Part model, mm, in its own coordinate system. A direction names the side the tool comes from. Coordinates: 2 decimals unless noted, no trailing zeros. Order: outer loops, then holes, each group sorted by start corner. A loop starts at its lowest first (then second) coordinate and runs counter-clockwise, first axis right, second up.
1) Cut at B-B (x = 0). List the corners of the cut face in (y, z).
2) Cut at C-C (y = 13.5). List the corners of the cut face in (x, z), and give its area (3 significant figures).
3) Wall check: L1, parallel to X at y = -3.3, z = 0; L2, parallel to Z at x = 7.5, y = -1.05; L3, parallel to Y at x = 9, z = 2.75. Give the ranges that are in metal, low to high.
4) Tool access for faces 4 (the cylindrical face through (1.43, -45.14, -2.75)), 5 (the flat face through (7.66, -45.87, 1.51)), 6 (the flat face through (0, 10, -1.5)), 7 (the cylindrical face through (6.25, -2.46, -0.05)): list every direction of +Z, -Z, +X, -X, +Y, -Y with a clear straight run to the whole face (end or side of a thin tool).
5) Cut at D-D (z = -5.25). List the corners of the cut face in (x, y).
6) Mould opens along X. For faces 1 (the cylindrical face through (0, -49, -1)), 2 (the flat face through (-7.53, -45.875, -1.783)), 3 (the cylindrical face through (10.2, -31.4, -0.1)) say: +X half, -X half, draft (parallel to the pull), parting line (faces both ways), or undercut.
7) Pin check, flat tips, straight feed: pin 1 Ø3 at (x, z) = (7.5, 0) entering from -Y; pin 2 Ø10.5 at (x, y) = (3, -28) entering from -Z; pin 3 Ø6 at (x, z) = (-5, -6) entering from -Y; pin 4 Ø6 at (x, z) = (4.5, -2) entering from +Y. Stop position of each tip, or through.
```python
from build123d import *

# Parameters (mm, degrees)
SKETCH_R              = 10
PAD_DEPTH             = 19
SKETCH001_R           = 3.5
PAD001_DEPTH          = 3
SKETCH002_R           = 2
PAD002_DEPTH          = 14.5
SKETCH003_W           = 10
SKETCH003_H           = 5
POCKET_DEPTH          = 14.5
PAD003_DEPTH          = 25.1
SKETCH005_R           = 3.1
PAD004_DEPTH          = 2.1
SKETCH006_R           = 1
PAD005_DEPTH          = 6
PAD006_DEPTH          = 3.6
SKETCH009_R           = 0.5
POCKET001_DEPTH       = 5
POLARPATTERN_COUNT    = 2
POLARPATTERN001_COUNT = 2
SKETCH010_R           = 1.25
POCKET002_DEPTH       = 5


with BuildPart() as part:
    # Sketch → Pad (new body)
    with BuildSketch(Plane.XZ):
        Circle(SKETCH_R)
    extrude(amount=PAD_DEPTH)

    # Sketch001 (on Face2 of Pad) → Pad001 (join)
    with BuildSketch(Plane(origin=(0, 0, 0), x_dir=(1, 0, 0), z_dir=(0, 1, 0))):
        Circle(SKETCH001_R)
    extrude(amount=PAD001_DEPTH)

    # Sketch002 (on Face5 of Pad001) → Pad002 (join)
    with BuildSketch(Plane(origin=(0, 3, 0), x_dir=(1, 0, 0), z_dir=(0, 1, 0))):
        Circle(SKETCH002_R)
    extrude(amount=PAD002_DEPTH)

    # Sketch003 (on Face7 of Pad002) → Pocket (cut)
    with BuildSketch(Plane(origin=(0, 17.5, 0), x_dir=(1, 0, 0), z_dir=(0, 1, 0))):
        with Locations((0, 4)):
            Rectangle(SKETCH003_W, SKETCH003_H)
    extrude(amount=-POCKET_DEPTH, mode=Mode.SUBTRACT)

    # Sketch004 (on Face3 of Pocket) → Pad003 (join)
    with BuildSketch(Plane.XZ.offset(19)):
        with BuildLine():
            Line((-6.689544, 7.7), (6.689544, 7.7))
            ThreePointArc((6.689544, -7.7), (10.2, 0), (6.689544, 7.7))
            Line((6.689544, -7.7), (-6.689544, -7.7))
            ThreePointArc((-6.689544, 7.7), (-10.2, 0), (-6.689544, -7.7))
        make_face()
    extrude(amount=PAD003_DEPTH)

    # Sketch005 (on Face14 of Pad003) → Pad004 (join)
    with BuildSketch(Plane.XZ.offset(44.1)):
        Circle(SKETCH005_R)
    extrude(amount=PAD004_DEPTH)

    # Sketch006 (on Face21 of Pad004) → Pad005 (join)
    with BuildSketch(Plane.XZ.offset(46.2)):
        Circle(SKETCH006_R)
    extrude(amount=PAD005_DEPTH)

    # Sketch008 (on Face14 of Pad005) → Pad006 (join)
    with BuildSketch(Plane.XZ.offset(44.1)):
        Polygon((6.603759, 1.445812), (8.483144, 2.129852), (8.58575, 1.847944), (6.706365, 1.163904), align=None)
    pad006 = extrude(amount=PAD006_DEPTH)

    # Sketch009 (on Face21 of Pad006) → Pocket001 (cut)
    with BuildSketch(Plane(origin=(0.410424, 0, -1.127631), x_dir=(0.939693, 0, 0.34202), z_dir=(0.34202, 0, -0.939693))):
        with Locations((7.689708, 46.695641)):
            Circle(SKETCH009_R)
    pocket001 = extrude(amount=-POCKET001_DEPTH, mode=Mode.SUBTRACT)

    # PolarPattern: Pad006 ×2 about axis
    polarpattern_axis = Axis((0, -44.1, 0), (0, -1, 0))
    for i in range(1, POLARPATTERN_COUNT):
        add(pad006.rotate(polarpattern_axis, i * 360 / POLARPATTERN_COUNT))

    # PolarPattern001: Pocket001 ×2 about axis
    polarpattern001_axis = Axis((0, 0, 0), (0, 1, 0))
    for i in range(1, POLARPATTERN001_COUNT):
        add(pocket001.rotate(polarpattern001_axis, i * 360 / POLARPATTERN001_COUNT), mode=Mode.SUBTRACT)

    # Sketch010 (on Face2 of PolarPattern001) → Pocket002 (cut)
    with BuildSketch(Plane(origin=(0, 0, 0), x_dir=(1, 0, 0), z_dir=(0, 1, 0))):
        with Locations((7.5, 0)):
            Circle(SKETCH010_R)
        with Locations((-7.5, 0)):
            Circle(SKETCH010_R)
    extrude(amount=-POCKET002_DEPTH, mode=Mode.SUBTRACT)


solid = part.part
```
Geometry check:
1. outline: (-52.2, -1) - (-46.2, -1) - (-46.2, -3.1) - (-44.1, -3.1) - (-44.1, -7.7) - (-19, -7.7) - (-19, -10) - (0, -10) - (0, -3.5) - (3, -3.5) - (3, -1.5) - (17.5, -1.5) - (17.5, 2) - (3, 2) - (3, 3.5) - (0, 3.5) - (0, 10) - (-19, 10) - (-19, 7.7) - (-44.1, 7.7) - (-44.1, 3.1) - (-46.2, 3.1) - (-46.2, 1) - (-52.2, 1) - close
2. outline: (-1.32, -1.5) - (1.32, -1.5) arc R2 ccw (long way) to start
2. area: 11.7 mm2
3. L1: x = -10 to -8.75, -6.25 to 6.25, 8.75 to 10
3. L2: z = -6.61 to -1.25, 1.25 to 6.61
3. L3: y = -44.1 to 0
4. face 4: -Y
4. face 5: -Z, +X, -Y
4. face 6: -Z, +X, -X, +Y
4. face 7: +Y
5. outline: (-8.75, -44.1) - (8.75, -44.1) - (8.75, -19) - (8.51, -19) - (8.51, 0) - (-8.51, 0) - (-8.51, -19) - (-8.75, -19) - close
6. face 1: parting line
6. face 2: undercut
6. face 3: +X half
7. pin 1: stops at y = -47.7
7. pin 2: stops at z = -7.7
7. pin 3: stops at y = -44.1
7. pin 4: stops at y = 17.5
